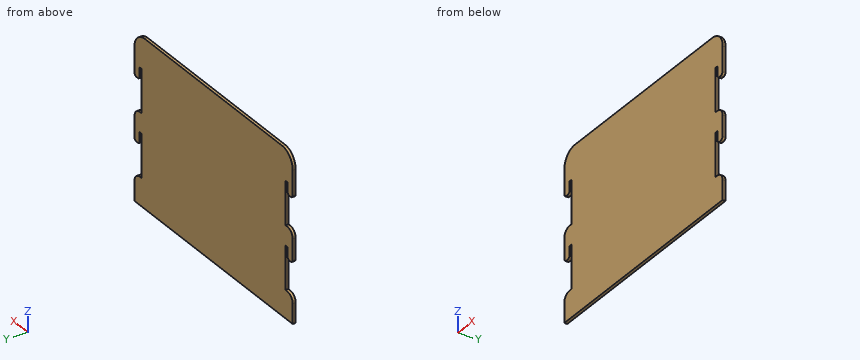
```python
from build123d import *

# Parameters (mm, degrees)
F1_DEPTH = 19.05
F2_W     = 19.05
F2_H     = 279.4
F3_DEPTH = 19.051


with BuildPart() as f1:
    # F0 (on Front) → F1 (new body)
    with BuildSketch(Plane.XZ):
        with BuildLine():
            Line((-743.168125, 218.486937), (-730.468125, 218.486937))
            ThreePointArc((-730.468125, 218.486937), (-716.99774, 224.066552), (-711.418125, 237.536937))
            Line((-711.418125, 237.536937), (-711.418125, 15.286937))
            ThreePointArc((-711.418125, 15.286937), (-747.339149, 0.407961), (-762.218125, -35.513063))
            Line((-762.218125, -35.513063), (-762.218125, -168.863063))
            ThreePointArc((-762.218125, -168.863063), (-756.638509, -182.333448), (-743.168125, -187.913063))
            Line((-743.168125, -187.913063), (-730.468125, -187.913063))
            ThreePointArc((-730.468125, -187.913063), (-716.99774, -182.333448), (-711.418125, -168.863063))
            Line((-711.418125, -168.863063), (-711.418125, -391.113063))
            ThreePointArc((-711.418125, -391.113063), (-747.339149, -405.992039), (-762.218125, -441.913063))
            Line((-762.218125, -441.913063), (-762.218125, -568.913063))
            Line((-762.218125, -568.913063), (-711.418125, -568.913063))
            Line((-711.418125, -568.913063), (-692.368125, -568.913063))
            Line((-692.368125, -568.913063), (691.931875, -568.913063))
            Line((691.931875, -568.913063), (710.981875, -568.913063))
            Line((710.981875, -568.913063), (761.781875, -568.913063))
            Line((761.781875, -568.913063), (761.781875, -441.913063))
            ThreePointArc((761.781875, -441.913063), (746.9029, -405.992039), (710.981875, -391.113063))
            Line((710.981875, -391.113063), (710.981875, -168.863063))
            ThreePointArc((710.981875, -168.863063), (716.561491, -182.333448), (730.031875, -187.913063))
            Line((730.031875, -187.913063), (742.731875, -187.913063))
            ThreePointArc((742.731875, -187.913063), (756.20226, -182.333448), (761.781875, -168.863063))
            Line((761.781875, -168.863063), (761.781875, -35.513063))
            ThreePointArc((761.781875, -35.513063), (746.9029, 0.407961), (710.981875, 15.286937))
            Line((710.981875, 15.286937), (710.981875, 237.536937))
            ThreePointArc((710.981875, 237.536937), (716.561491, 224.066552), (730.031875, 218.486937))
            Line((730.031875, 218.486937), (742.731875, 218.486937))
            ThreePointArc((742.731875, 218.486937), (756.20226, 224.066552), (761.781875, 237.536937))
            Line((761.781875, 237.536937), (763.606541, 395.110511))
            ThreePointArc((763.606541, 395.110511), (734.270133, 467.711845), (662.013352, 497.886937))
            Line((662.013352, 497.886937), (-660.618125, 497.886937))
            ThreePointArc((-660.618125, 497.886937), (-732.460174, 468.128986), (-762.218125, 396.286937))
            Line((-762.218125, 396.286937), (-762.218125, 237.536937))
            ThreePointArc((-762.218125, 237.536937), (-756.638509, 224.066552), (-743.168125, 218.486937))
        make_face()
    extrude(amount=F1_DEPTH)

    # F2 (on face) → F3 (cut, through all)
    with BuildSketch(Plane.XZ.offset(19.05)):
        with Locations((-701.893125, 154.986937)):
            Rectangle(F2_W, F2_H)
        with Locations((-701.893125, -251.413063)):
            Rectangle(F2_W, F2_H)
        with Locations((701.893125, 154.986937)):
            Rectangle(F2_W, F2_H)
        with Locations((701.893125, -251.413063)):
            Rectangle(F2_W, F2_H)
    extrude(amount=-F3_DEPTH, mode=Mode.SUBTRACT)


solid = f1.part
```
The model under review builds one solid part; all positions refer to its coordinate system, in mm. Give positions to 0.01 mm unless a question says otherwise; leave off trailing zeros. Loops run counter-clockwise (first coordinate to the right, second up) from the corner with the lowest first, then second, coordinate; pieces in that order, holes last. Notation, with made-up numbers: (-38.5, 73.5) - (12.5, 73.5) arc R31 cw to (12.5, 104.5) - close; hole circle Ø5 at (-31.5, 64.5). An arc over 180 degrees is marked (long way). Answer as a JSON object with one key per item and string values.
Q1. Insertion check: pin 1 (2 mm diameter, centred on y = -15.5, z = 304, fed in from +X); pin 2 (8 mm diameter, centred on y = -15, z = -460, fed in from +X); pin 3 (9.5 mm diameter, centred on x = -700.5, y = -13, fed in from +Z). Each pin has a flat end and moves straight along its axis. Give the tip position at first contact, or say it passes through.
Worked out:
{"pin 1": "stops at x = 762.56", "pin 2": "stops at x = 761.78", "pin 3": "stops at z = 491.62"}
Q2. Add section A-A on z = -285. State the section outline as (x, y) points.
Worked out:
{"outline": "(-692.37, -19.05) - (692.37, -19.05) - (692.37, 0) - (-692.37, 0) - close"}
Q3. To check wall thickness, follow line 1 along Z through (x, y) = (-699.5, -6.5); line 2 along X through (y, z) = (-6.25, -178); line 3 along X through (y, z) = (-13, -47.5). State the ranges of each line that lie inside material, in increasing order.
Worked out:
{"line 1": "z = -568.91 to -391.11, -111.71 to 15.29, 294.69 to 490.15", "line 2": "x = -759.88 to -713.75, -692.37 to 692.37, 713.32 to 759.45", "line 3": "x = -762.22 to 761.78"}
